Source: CAD feature listing. Evaluate the final solid. Frame: model axes, mm. A direction names the side the tool comes from. Give positions to 0.01 mm unless a question says otherwise; leave off trailing zeros. Loops run counter-clockwise (first coordinate to the right, second up) from the corner with the lowest first, then second, coordinate; pieces in that order, holes last. Notation, with made-up numbers: M -6.75,-19.5 L 29.25,-19.5 A14 ccw 29.25,-10.5 Z; hole C -2,20 d7. An arc over 180 degrees is marked long. Put each result on its own line as item: value.
from build123d import *

# Parameters (mm, degrees)
SKETCH2_R               = 38.1
BOSS_EXTRUDE1_DEPTH     = 12.7
SKETCH3_R               = 19.05
BOSS_EXTRUDE2_DEPTH     = 101.6
SKETCH4_W               = 30.48
SKETCH4_H               = 12.7
BOSS_EXTRUDE3_DEPTH     = 50.8
FILLET1_R               = 6.35
SKETCH5_R               = 12.7
CUT_EXTRUDE1_DEPTH      = 32.75
CUT_EXTRUDE1_DEPTH_BACK = 45.45


with BuildPart() as part:
    # Sketch2 → Boss-Extrude1 (new body, symmetric)
    with BuildSketch(Plane.XY):
        Circle(SKETCH2_R)
    extrude(amount=BOSS_EXTRUDE1_DEPTH, both=True)

    # Sketch3 → Boss-Extrude2 (add)
    with BuildSketch(Plane.XY.offset(12.7)):
        Circle(SKETCH3_R)
    extrude(amount=BOSS_EXTRUDE2_DEPTH)

    # Sketch4 → Boss-Extrude3 (add)
    with BuildSketch(Plane.XY.offset(114.3)):
        Rectangle(SKETCH4_W, SKETCH4_H)
    extrude(amount=BOSS_EXTRUDE3_DEPTH)

    # Fillet1
    fillet1_edges = [part.edges().sort_by_distance(p)[0] for p in [
        (15.24, 0, 165.1),
        (-15.24, 0, 165.1),
    ]]
    fillet(fillet1_edges, radius=FILLET1_R)

    # Sketch5 → Cut-Extrude1 (cut, two sides)
    with BuildSketch(Plane(origin=(0, 6.35, 0), x_dir=(1, 0, 0), z_dir=(0, 1, 0))) as cut_extrude1_sk:
        with Locations((0, -139.7)):
            Circle(SKETCH5_R)
    extrude(amount=CUT_EXTRUDE1_DEPTH, mode=Mode.SUBTRACT)
    extrude(cut_extrude1_sk.sketch, amount=-CUT_EXTRUDE1_DEPTH_BACK, mode=Mode.SUBTRACT)


solid = part.part
1. Section query D-D (z = 76). Output: boundary loops of the cut face in (x, y).
Found:
outline: C 0,0 d38.1
2. Draft query along X for faces 1 (the cylindrical face through (-2.75, 0.09, 152.1)), 2 (the cylindrical face through (13.43, 0.09, 163.19)), 3 (the flat face through (7, -6.35, 128)), 4 (the cylindrical face through (-15.12, -11.59, 62.79)). Return one class per face: pulls with the +X half, pulls with the -X half, needs draft (parallel to the pull), parting line crosses it, or undercut.
Found:
face 1: undercut
face 2: pulls with the +X half
face 3: needs draft
face 4: parting line crosses it
3. Section query B-B (z = 143). Output: boundary loops of the cut face in (x, y), plus the area to 3 significant figures.
Found:
outline: M -15.24,-6.35 L -12.26,-6.35 L -12.26,6.35 L -15.24,6.35 Z; M 12.26,-6.35 L 15.24,-6.35 L 15.24,6.35 L 12.26,6.35 Z
area: 75.6 mm^2
4. Contact query for flat-ended pins moving along their axis: P1, Ø12, axis at x = 23.5, z = 28.5, coming from the +Y side; P2, Ø10, axis at x = -17, y = -3.5, coming from the +Z side; P3, Ø10, axis at y = -21.5, z = 53.5, coming from the +X side. Output: stop coordinate, or through.
Found:
P1: y = 7.53
P2: z = 164.29
P3: x = 9.52
5. Material intervals for line 1 (X direction, y = -3, z = 139.7); line 2 (Z direction, x = 0, y = 1.75); line 3 (Y direction, x = 13.5, z = 139.5), sorted ascending. Write a range as from..to.
Found:
line 1: -15.24..-12.7, 12.7..15.24
line 2: -12.7..127, 152.4..165.1
line 3: -6.35..6.35
6. Section query A-A (x = 0). Output: boundary loops of the cut face in (y, z).
Found:
outline: M -38.1,-12.7 L 38.1,-12.7 L 38.1,12.7 L 19.05,12.7 L 19.05,114.3 L 6.35,114.3 L 6.35,127 L -6.35,127 L -6.35,114.3 L -19.05,114.3 L -19.05,12.7 L -38.1,12.7 Z; M -6.35,152.4 L 6.35,152.4 L 6.35,165.1 L -6.35,165.1 Z
7. Access query for faces 5 (the flat face through (-15.24, 0, 136)), 6 (the flat face through (7, 6.35, 128)), 7 (the flat face through (7.9, 17.5, 12.7)), 8 (the flat face through (15.24, 0, 136)). Directions: +Z, -Z, +X, -X, +Y, -Y. A direction counts if a zero-diameter tool reaches every point of the face in a straight line with its end or side. Return the directions, or none.
Found:
face 5: +Z, -X, +Y, -Y
face 6: +Z, +X, -X, +Y
face 7: +Z
face 8: +Z, +X, +Y, -Y
8. Section query C-C (y = 0). Output: boundary loops of the cut face in (x, z), plus the area to 3 significant figures.
Found:
outline: M -38.1,-12.7 L 38.1,-12.7 L 38.1,12.7 L 19.05,12.7 L 19.05,114.3 L 15.24,114.3 L 15.24,158.75 A6.35 ccw 8.89,165.1 L -8.89,165.1 A6.35 ccw -15.24,158.75 L -15.24,114.3 L -19.05,114.3 L -19.05,12.7 L -38.1,12.7 Z; hole C 0,139.7 d25.4
area: 6,830 mm^2
